```python
from build123d import *

# Parameters (mm, degrees)
SKETCH_R         = 10.15
SKETCH_R_2       = 1.675
PAD_DEPTH        = 8
SKETCH001_R      = 18.5
POCKET_DEPTH     = 7
POCKET001_DEPTH  = 1.6
POCKET004_DEPTH  = 3
CHAMFER_SIZE     = 2
POCKET002_DEPTH  = 7.4
SKETCH005_R      = 10.775
SKETCH005_R_2    = 10.15
PAD001_DEPTH     = 5.1
CHAMFER001_ANGLE = 64
CHAMFER001_SIZE  = 2.9
CHAMFER002_ANGLE = 60
CHAMFER002_SIZE  = 2.9
FILLET_R         = 6


with BuildPart() as part:
    # Sketch → Pad (new body)
    with BuildSketch(Plane.XY):
        Polygon((0, 37.5), (37.5, 0), (0, -37.5), (-37.5, 0), align=None)
        Circle(SKETCH_R, mode=Mode.SUBTRACT)
        with Locations((0, 30)):
            Circle(SKETCH_R_2, mode=Mode.SUBTRACT)
        with Locations((30, 0)):
            Circle(SKETCH_R_2, mode=Mode.SUBTRACT)
        with Locations((0, -30)):
            Circle(SKETCH_R_2, mode=Mode.SUBTRACT)
        with Locations((-30, 0)):
            Circle(SKETCH_R_2, mode=Mode.SUBTRACT)
    extrude(amount=-PAD_DEPTH)

    # Sketch001 → Pocket (cut)
    with BuildSketch(Plane.XY):
        Circle(SKETCH001_R)
    extrude(amount=-POCKET_DEPTH, mode=Mode.SUBTRACT)

    # Sketch002 → Pocket001 (cut)
    with BuildSketch(Plane.XY):
        with BuildLine():
            Line((-16.846352, 11.236678), (-17.67827, 11.791576))
            ThreePointArc((-11.732099, 17.717798), (-15.000749, 15.051247), (-17.67827, 11.791576))
            Line((-11.18, 16.884019), (-11.732099, 17.717798))
            ThreePointArc((16.897228, -11.160027), (14.310444, 14.327376), (-11.18, 16.884019))
            Line((16.897228, -11.160027), (17.731659, -11.711139))
            ThreePointArc((11.812473, -17.664314), (15.068975, -14.98294), (17.731659, -11.711139))
            Line((11.256591, -16.833052), (11.812473, -17.664314))
            ThreePointArc((-11.17334, -16.888427), (0.049993, -20.249938), (11.256591, -16.833052))
            Line((-11.17334, -16.888427), (-11.72511, -17.722423))
            ThreePointArc((-17.673618, -11.798547), (-14.994812, -15.057162), (-11.72511, -17.722423))
            Line((-16.841919, -11.243321), (-17.673618, -11.798547))
            ThreePointArc((-16.846352, 11.236678), (-20.25, -0.003993), (-16.841919, -11.243321))
        make_face()
    extrude(amount=-POCKET001_DEPTH, mode=Mode.SUBTRACT)

    # Sketch004 → Pocket004 (cut)
    with BuildSketch(Plane.XY):
        with BuildLine():
            Line((3.47625, 19.949391), (3.09, 17.732792))
            ThreePointArc((8.300497, 15.971905), (5.762902, 17.052535), (3.09, 17.732792))
            Line((8.300497, 15.971905), (9.338059, 17.968393))
            ThreePointArc((9.338059, 17.968393), (6.483264, 19.184102), (3.47625, 19.949391))
        make_face()
    extrude(amount=-POCKET004_DEPTH, mode=Mode.SUBTRACT)

    # Chamfer
    chamfer_edges = [part.edges().sort_by_distance(p)[0] for p in [
        (18.75, -18.75, -8),
        (37.5, 0, -4),
        (0, -37.5, -4),
        (-18.75, -18.75, -8),
        (-37.5, 0, -4),
        (-18.75, 18.75, -8),
        (0, 37.5, -4),
        (18.75, 18.75, -8),
    ]]
    chamfer(chamfer_edges, length=CHAMFER_SIZE)

    # Sketch003 → Pocket002 (cut)
    with BuildSketch(Plane.XY):
        Polygon((7.071068, 15.909903), (15.909903, 7.071068), (26.516504, 17.67767), (17.67767, 26.516504), align=None)
    extrude(amount=-POCKET002_DEPTH, mode=Mode.SUBTRACT)

    # Sketch005 (on DatumPlane) → Pad001 (join)
    with BuildSketch(Plane.XY.offset(-7)):
        Circle(SKETCH005_R)
        Circle(SKETCH005_R_2, mode=Mode.SUBTRACT)
    extrude(amount=PAD001_DEPTH)

    # Chamfer001
    chamfer001_edges = [part.edges().sort_by_distance(p)[0] for p in [
        (-10.15, 0, -8),
    ]]
    chamfer001_side = part.faces().sort_by_distance((16.642355, -16.642355, -8))[0]
    chamfer(chamfer001_edges, length=CHAMFER001_SIZE, angle=CHAMFER001_ANGLE, reference=chamfer001_side)

    # Chamfer002
    chamfer002_edges = [part.edges().sort_by_distance(p)[0] for p in [
        (-10.775, 0, -7),
    ]]
    chamfer002_side = part.faces().sort_by_distance((-15.182869, -9.62516, -7))[0]
    chamfer(chamfer002_edges, length=CHAMFER002_SIZE, angle=CHAMFER002_ANGLE, reference=chamfer002_side)

    # Fillet
    fillet_edges = [part.edges().sort_by_distance(p)[0] for p in [
        (-13.05, 0, -8),
        (-13.675, 0, -7),
    ]]
    fillet(fillet_edges, radius=FILLET_R)


solid = part.part
```
Can you work these out from the model? Positions are in its coordinate system, mm. A direction names the side the tool comes from. Give positions to 0.01 mm unless a question says otherwise; leave off trailing zeros. Loops run counter-clockwise (first coordinate to the right, second up) from the corner with the lowest first, then second, coordinate; pieces in that order, holes last. Notation, with made-up numbers: M -0.75,-20.75 L 3.25,-20.75 A20 cw 3.25,18.25 Z; hole C -15,24 d10. An arc over 180 degrees is marked long. One line per item, written item: value.
(1) Suppose I cut it at C-C on y = -21.5. List the corners of the cut face in (x, z) for me.
Returned:
outline: M -16,-6 L -13.17,-8 L 13.17,-8 L 16,-6 L 16,0 L -16,0 Z
(2) Which directions (+Z, -Z, +X, -X, +Y, -Y) give clear straight access to the entire face, cutting with the end or side of a thin tool? Please do faces 5 (the face through (-28.45, -0.64, -3.94)), 6 (the face through (-0.12, -20.25, -0.79)).
Returned:
face 5: +Z, -Z
face 6: +Z
(3) Will these pins go through, and if not, where does the flat tip stop? pin 1 (3 mm diameter, centred on x = 19, y = 0.5, fed in from +Z); pin 2 (4 mm diameter, centred on x = 24.5, z = -4.5, fed in from -Y); pin 3 (2.5 mm diameter, centred on x = 5, y = 18, fed in from +Z); pin 4 (1 mm diameter, centred on x = -20.5, z = -4.5, fed in from -Y).
Returned:
pin 1: z = 0
pin 2: y = -15
pin 3: z = -3
pin 4: y = -17.5
(4) We'd pull the mould along Y, two halves only. Please class faces 1 (the face through (16, 8, -8)), 2 (the face through (-5.6, -16.4, -7)), 3 (the face through (-18.5, -19, -3)), 4 (the face through (-18.295, 17.81, -6.986)): released by +Y, released by -Y, zero draft, split by the parting line, or undercut.
Returned:
face 1: zero draft
face 2: undercut
face 3: released by -Y
face 4: released by +Y
(5) Suppose I cut it at A-A on x = -30. List the corners of the cut face in (y, z) for me (3 decimals), plus the area to 3 significant figures.
Returned:
outline: M -7.5,-6 L -4.672,-8 L -1.675,-8 L -1.675,0 L -7.5,0 Z; M 1.675,-8 L 4.672,-8 L 7.5,-6 L 7.5,0 L 1.675,0 Z
area: 87.5 mm^2
(6) I need wall thicknesses on line 1 (Y direction, x = 0, z = -1.95) (3 decimals); line 2 (Y direction, x = -3, z = -3.75); line 3 (Y direction, x = -7, z = -3.75). Which ranges of each line are inside material? Lowest first, please.
Returned:
line 1: -36.086 to -31.675, -28.325 to -18.5, -10.775 to -10.15, 10.15 to 10.775, 18.5 to 28.325, 31.675 to 36.086
line 2: -34.5 to -18.26, -11.41 to -10.56, 10.56 to 11.41, 18.26 to 34.5
line 3: -30.5 to -17.12, -9.5 to -8.46, 8.46 to 9.5, 17.12 to 30.5
